```python
from build123d import *

# Parameters (mm, degrees)
F1_DEPTH  = 63.5
F2_DEPTH  = 50.8
F3_DEPTH  = 7.9375
F2_FACE_W = 50.8
F2_FACE_H = 28.575
F5_R      = 6.35


with BuildPart() as f1:
    # F0 (on Front) → F1 (new body, symmetric)
    with BuildSketch(Plane.XZ):
        Polygon((-41.275, 9.525), (-41.275, -9.525), (41.275, -9.525), (41.275, 9.525), (22.225, 9.525), align=None)
    extrude(amount=F1_DEPTH, both=True)

    # F0 (on Front) → F2 (join)
    with BuildSketch(Plane.XZ):
        with BuildLine():
            Line((22.225, 9.525), (41.275, 9.525))
            Line((41.275, 9.525), (41.275, 27.0002))
            ThreePointArc((41.275, 27.0002), (45.92468, 38.22552), (57.15, 42.8752))
            Line((57.15, 42.8752), (60.430248, 42.8752))
            Line((60.430248, 42.8752), (60.430248, 61.9252))
            Line((60.430248, 61.9252), (57.15, 61.9252))
            ThreePointArc((57.15, 61.9252), (32.454296, 51.695904), (22.225, 27.0002))
            Line((22.225, 27.0002), (22.225, 9.525))
        make_face()
        Polygon((60.430248, 66.675), (60.430248, 61.9252), (60.430248, 42.8752), (60.430248, 38.1), (85.830248, 38.1), (85.830248, 66.675), align=None)
    extrude(amount=F2_DEPTH)

    # F0 (on Front) → F3 (join, symmetric)
    with BuildSketch(Plane.XZ):
        with BuildLine():
            add(Edge.make_bspline(
                [(-41.275, 9.525), (-28.744785, 49.276773), (25.011688, 69.808759), (57.15, 61.9252)],
                knots=[0, 0, 0, 0, 111.504536, 111.504536, 111.504536, 111.504536], degree=3))
            Line((-41.275, 9.525), (22.225, 9.525))
            Line((22.225, 9.525), (22.225, 27.0002))
            ThreePointArc((22.225, 27.0002), (32.454296, 51.695904), (57.15, 61.9252))
        make_face()
    extrude(amount=F3_DEPTH, both=True)

    # F2_face (on face) → F4 (revolve)
    with BuildSketch(Plane(origin=(85.830248, -25.4, 52.3875), x_dir=(0, 1, 0), z_dir=(1, 0, 0))):
        Rectangle(F2_FACE_W, F2_FACE_H)
    revolve(axis=Axis((85.830248, 0, 52.3875), (0, 0, 1)))

    # F5
    f5_edges = [f1.edges().sort_by_distance(p)[0] for p in [
        (41.275, -63.5, 0),
        (-41.275, -63.5, 0),
        (41.275, 63.5, 0),
        (-41.275, 63.5, 0),
    ]]
    fillet(f5_edges, radius=F5_R)


solid = f1.part
```
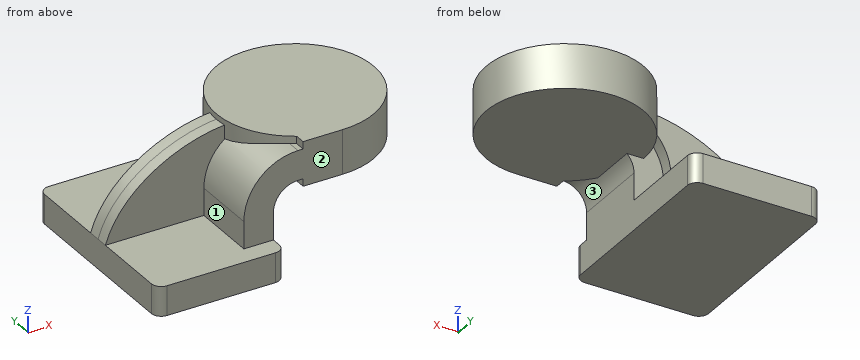
Part model, mm, in its own coordinate system. Face numbers are marked on the shaded views. A direction names the side the tool comes from. Give positions to 0.01 mm unless a question says otherwise; leave off trailing zeros. Order: outer loops, then holes, each group sorted by start corner. A loop starts at its lowest first (then second) coordinate and runs counter-clockwise, first axis right, second up. Notation, with made-up numbers: M -18.75,45 L 17.25,45 A25 cw 17.25,60 Z; hole C -37,-9.5 d10. An arc over 180 degrees is marked long. Use a Markdown table: item, result. Add a question column.
(1) Drop flat-ended pins along their axis: P1, Ø5, axis at x = 18, z = 42.5, coming from the -Y side; P2, Ø4, axis at x = 46, y = -0.5, coming from the -Z side; P3, Ø2.5, axis at y = -46, z = 63.5, coming from the -X side. Give the stop position or say it passes through.
(2) Saw through at A-A, the plane z = 5.5. Give the cut face in (x, y) (3 decimals), and give its area (3 significant figures).
(3) Saw through at C-C, the plane x = 89.5. Give the cut face in (y, z) (3 decimals).
(4) Saw through at B-B, the plane y = -15.5. Give the cut face in (x, z) (3 decimals), and give its area (3 significant figures).
(5) Probe line 1 along X through (y, z) = (-46.5, 22.5) (3 decimals); line 2 along Z through (x, y) = (-31, 58) (3 decimals); line 3 along Z through (x, y) = (105.5, -34) (3 decimals). List the from-to ranges inside material, lowest first. Write a range as [from, to].
(6) 3-axis set-ups, long thin cutter, end or side, ignore diameter. For the marked faces 1, 2 and 3: which of +Z, -Z, +X, -X, +Y, -Y reach the whole face in a straight line?
Answer key:
| question | item | result |
|---|---|---|
| 1 | P1 | y = -7.94 |
| 1 | P2 | z = 35.89 |
| 1 | P3 | x = 60.43 |
| 2 | outline | M -41.275,-57.15 A6.35 ccw -34.925,-63.5 L 34.925,-63.5 A6.35 ccw 41.275,-57.15 L 41.275,57.15 A6.35 ccw 34.925,63.5 L -34.925,63.5 A6.35 ccw -41.275,57.15 Z |
| 2 | area | 10,400 mm^2 |
| 3 | outline | M -50.667,38.1 L 50.667,38.1 L 50.667,66.675 L -50.667,66.675 Z |
| 4 | outline | M -41.275,-9.525 L 41.275,-9.525 L 41.275,27 A15.875 cw 45.801,38.1 L 134.208,38.1 L 134.208,66.675 L 37.453,66.675 L 37.453,55.841 A34.925 ccw 22.225,27 L 22.225,9.525 L -41.275,9.525 Z |
| 4 | area | 5,040 mm^2 |
| 5 | line 1 | [22.225, 41.275] |
| 5 | line 2 | [-9.525, 9.525] |
| 5 | line 3 | [38.1, 66.675] |
| 6 | face 1 | +Z, -X, -Y |
| 6 | face 2 | +Z, +X, -X, -Y |
| 6 | face 3 | -Z, -Y |
